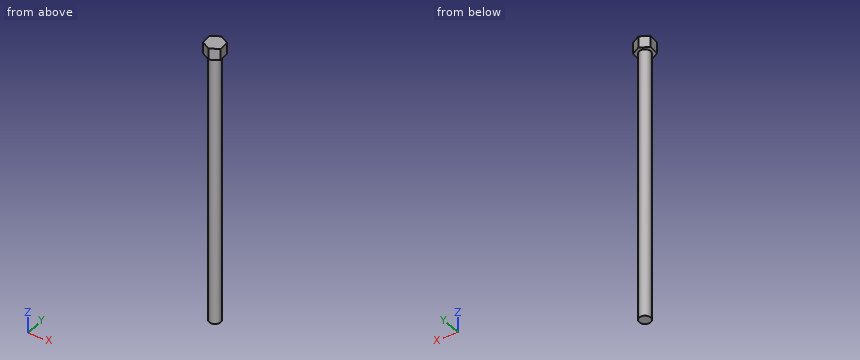
```python
from build123d import *

# Parameters (mm, degrees)
F0_R     = 4
F1_DEPTH = 200
F3_DEPTH = 8


with BuildPart() as f1:
    # F0 (on Top) → F1 (new body)
    with BuildSketch(Plane.XY):
        Circle(F0_R)
    extrude(amount=F1_DEPTH)

    # F2 (on face) → F3 (join)
    with BuildSketch(Plane.XY.offset(200)):
        Polygon((5.900696, 3.666764), (-0.225163, 6.943534), (-6.125859, 3.276771), (-5.900696, -3.666764), (0.225163, -6.943534), (6.125859, -3.276771), align=None)
    extrude(amount=-F3_DEPTH)


solid = f1.part
```
Work out the finished part from the listing and answer in its coordinate system (mm). Give positions to 0.01 mm unless a question says otherwise; leave off trailing zeros. Order: outer loops, then holes, each group sorted by start corner. A loop starts at its lowest first (then second) coordinate and runs counter-clockwise, first axis right, second up.
1. Each of these flat-tipped pins is pushed along its axis until it touches: P1, Ø8, axis at y = -1, z = 131, coming from the -X side; P2, Ø3, axis at x = -3.5, z = 69.5, coming from the +Y side; P3, Ø1, axis at y = 5.5, z = 172.5, coming from the +X side; P4, Ø4, axis at y = -4.5, z = 163.5, coming from the +X side. Where does it stop, or does it pass through?
Result sheet:
P1: stops at x = -4
P2: stops at y = 3.46
P3: passes through
P4: stops at x = 3.12
2. Section A-A, the plane y = 0 is taken. Determine the outline of the cut face in (x, z), and give its area (3 significant figures).
Result sheet:
outline: (-6.02, 192) - (-4, 192) - (-4, 0) - (4, 0) - (4, 192) - (6.02, 192) - (6.02, 200) - (-6.02, 200) - close
area: 1,630 mm2
3. Section B-B, the plane z = 60.5 is taken. Determine the outline of the cut face in (x, y), and give its area (3 significant figures).
Result sheet:
outline: circle Ø8 at (0, 0)
area: 50.3 mm2
4. Straight lines are drawn through the part: L1, parallel to X at y = -2.25, z = 23; L2, parallel to Y at x = 1.5, z = 157. For each, find the intervals that lie inside material, in ascending order.
Result sheet:
L1: x = -3.31 to 3.31
L2: y = -3.71 to 3.71
5. Section C-C, the plane x = 2 is taken. Determine the outline of the cut face in (y, z).
Result sheet:
outline: (-5.84, 192) - (-3.46, 192) - (-3.46, 0) - (3.46, 0) - (3.46, 192) - (5.75, 192) - (5.75, 200) - (-5.84, 200) - close
